Build history of the part. All positions in model axes, mm. Coordinates: 2 decimals unless noted, no trailing zeros. Order: outer loops, then holes, each group sorted by start corner. A loop starts at its lowest first (then second) coordinate and runs counter-clockwise, first axis right, second up. Notation, with made-up numbers: (56.25, 29) - (104.25, 29) arc R25 ccw to (104.25, 67) - close; hole circle Ø1 at (-38.5, 39). An arc over 180 degrees is marked (long way). One line per item, written item: value.
from build123d import *

# Parameters (mm, degrees)
SKETCH1_R           = 5
SKETCH1_R_2         = 1.5
BOSS_EXTRUDE1_DEPTH = 3


with BuildPart() as part:
    # Sketch1 → Boss-Extrude1 (new body)
    with BuildSketch(Plane.XY):
        with BuildLine():
            Line((121.815327096, 13.144873556), (146.959411549, -36.24203935))
            Line((146.959411549, -36.24203935), (146.959411549, -47.411715326))
            Line((146.959411549, -47.411715326), (2.561732102, -47.411715326))
            Line((2.561732102, -47.411715326), (-17.136179556, -8.72517889))
            ThreePointArc((-17.136179556, -8.72517889), (-10.596670935, 16.046431426), (14.753160039, 12.333761198))
            Line((14.753160039, 12.333761198), (121.815327096, 13.144873556))
        make_face()
        Circle(SKETCH1_R, mode=Mode.SUBTRACT)
        with Locations((12.609500958, 0)):
            Circle(SKETCH1_R_2, mode=Mode.SUBTRACT)
        with Locations((0, -12.609500958)):
            Circle(SKETCH1_R_2, mode=Mode.SUBTRACT)
        with Locations((-12.609500958, 0)):
            Circle(SKETCH1_R_2, mode=Mode.SUBTRACT)
        with Locations((0, 12.609500958)):
            Circle(SKETCH1_R_2, mode=Mode.SUBTRACT)
    extrude(amount=BOSS_EXTRUDE1_DEPTH)


solid = part.part
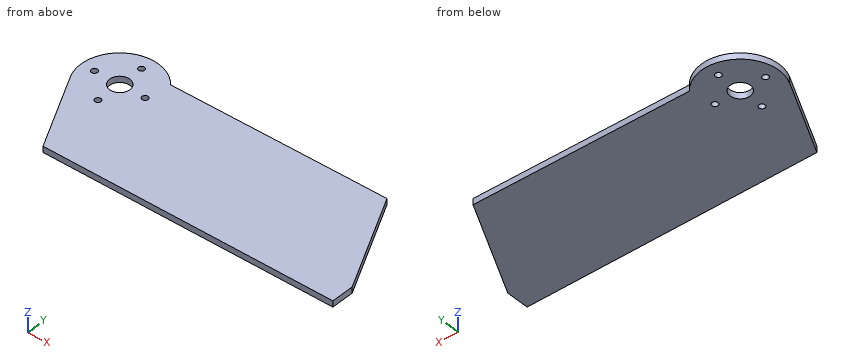
1. Probe line 1 along Y through (x, z) = (0, 1.6); line 2 along X through (y, z) = (3.5, 2.15); line 3 along X through (y, z) = (-44, 2.2). List the from-to ranges inside material, lowest first.
Values found:
line 1: y = -42.38 to -14.11, -11.11 to -5, 5 to 11.11, 14.11 to 19.23
line 2: x = -18.91 to -3.57, 3.57 to 126.73
line 3: x = 0.82 to 146.96
2. Band-saw the part on A-A, the plane y = 0. Give the cut face in (x, z).
Values found:
outline: (-19.23, 0) - (-14.11, 0) - (-14.11, 3) - (-19.23, 3) - close; (-11.11, 0) - (-5, 0) - (-5, 3) - (-11.11, 3) - close; (5, 0) - (11.11, 0) - (11.11, 3) - (5, 3) - close; (14.11, 0) - (128.51, 0) - (128.51, 3) - (14.11, 3) - close
3. Band-saw the part on D-D, the plane y = -25. Give the cut face in (x, z).
Values found:
outline: (-8.85, 0) - (141.24, 0) - (141.24, 3) - (-8.85, 3) - close
4. Flat gauge pins, fed straight in: P1, Ø1.8, axis at x = 0, y = 12.61, coming from the -Z side; P2, Ø2, axis at x = 75, y = -21, coming from the -Z side; P3, Ø1.5, axis at y = -17.5, z = 2.5, coming from the -X side. Where does each tip first touch, or does it go through?
Values found:
P1: passes through
P2: stops at z = 0
P3: stops at x = -13.05
5. Band-saw the part on B-B, the plane z = 1.45. Give the cut face in (x, y).
Values found:
outline: (-17.14, -8.73) - (2.56, -47.41) - (146.96, -47.41) - (146.96, -36.24) - (121.82, 13.14) - (14.75, 12.33) arc R19.23 ccw to start; hole circle Ø3 at (-12.61, 0); hole circle Ø10 at (0, 0); hole circle Ø3 at (0, -12.61); hole circle Ø3 at (0, 12.61); hole circle Ø3 at (12.61, 0)
6. Band-saw the part on C-C, the plane x = 0. Give the cut face in (y, z), and give its area (3 significant figures).
Values found:
outline: (-42.38, 0) - (-14.11, 0) - (-14.11, 3) - (-42.38, 3) - close; (-11.11, 0) - (-5, 0) - (-5, 3) - (-11.11, 3) - close; (5, 0) - (11.11, 0) - (11.11, 3) - (5, 3) - close; (14.11, 0) - (19.23, 0) - (19.23, 3) - (14.11, 3) - close
area: 137 mm2
